Work out the finished part from the listing and answer in its coordinate system (mm). Face numbers are marked on the shaded views. A direction names the side the tool comes from. Coordinates: 2 decimals unless noted, no trailing zeros. Order: outer loops, then holes, each group sorted by start corner. A loop starts at its lowest first (then second) coordinate and runs counter-clockwise, first axis right, second up. Notation, with made-up numbers: M 44,-7.75 L 65,-7.75 A30 ccw 65,15.25 Z; hole C -18.75,13 d6. An arc over 180 degrees is marked long. Write item = value, one per line. Start each with the question number.
Q1. Straight lines are drawn through the part: line 1 along Y through (x, z) = (5, -7.5); line 2 along Z through (x, y) = (16, 13.5); line 3 along X through (y, z) = (4, -13). For each, find the intervals that lie inside material, in ascending order.
Q2. Find section B-B on z = -16. Give the vertices of the cut face in (x, y), and give its area (3 significant figures).
Q3. Find section A-A on y = 13.5. Give the vertices of the cut face in (x, z), and give its area (3 significant figures).
Q4. Determine the mould class of the marked faces 1, 2, 3 and 4 for opening direction X: released by +X, released by -X, zero draft, split by the parting line, or undercut.
Q5. A tool of negligible diameter and unlimited length cuts with its end or side. For the marked faces 5, 6 and 7, from which of +Z, -Z, +X, -X, +Y, -Y can it reach the whole face along a straight path? Write none if from no direction.
Q6. Each of these flat-tipped pins is pushed along its axis until it touches: P1, Ø5, axis at x = -6.5, z = -9, coming from the +Y side; P2, Ø5, axis at y = -2, z = 10, coming from the -X side; P3, Ø4, axis at y = -2.5, z = -10.5, coming from the +X side. Where does it stop, or does it pass through?
```python
from build123d import *

# Parameters (mm, degrees)
F4_D     = 4.2
F5_D     = 6.8
F6_D     = 6.6
F8_D     = 20
F8_DEPTH = 20
F8_TIP   = 6.0086061903


with BuildPart() as f2:
    # F1 (on Right) → F2 (revolve)
    with BuildSketch(Plane.YZ):
        Polygon((0, 0), (-16, 0), (-16, -12), (-12, -12), (-12, -30), (0, -30), align=None)
        Polygon((-22, 5), (-22, 0), (-16, 0), (0, 0), (0, 15), (-18, 15), (-18, 5), align=None)
    revolve(axis=Axis((0, 0, -7.8081190586), (0, 0, -1)))

    # F4 (through all)
    with Locations(Plane(origin=(0, 0, -30), x_dir=(1, 0, 0), z_dir=(0, 0, -1))):
        with Locations((4.0257674055, 6.3279694055)):
            Hole(F4_D / 2)

    # F5 (through all)
    with Locations(Plane(origin=(0, 0, -30), x_dir=(1, 0, 0), z_dir=(0, 0, -1))):
        with Locations((-3.2813517626, 2.2875162535)):
            Hole(F5_D / 2)

    # F6 (through all)
    with Locations(Plane(origin=(0, 0, -30), x_dir=(1, 0, 0), z_dir=(0, 0, -1))):
        with Locations((5.4357488604, -3.9169674911)):
            Hole(F6_D / 2)

    # F8
    with Locations(Plane.XY.offset(15)):
        with Locations((-3.2813517626, -2.2875162535)):
            Hole(F8_D / 2, depth=F8_DEPTH)
            with Locations((0, 0, -(F8_DEPTH + F8_TIP / 2))):  # 118° drill point
                Cone(0, F8_D / 2, F8_TIP, mode=Mode.SUBTRACT)


solid = f2.part
```
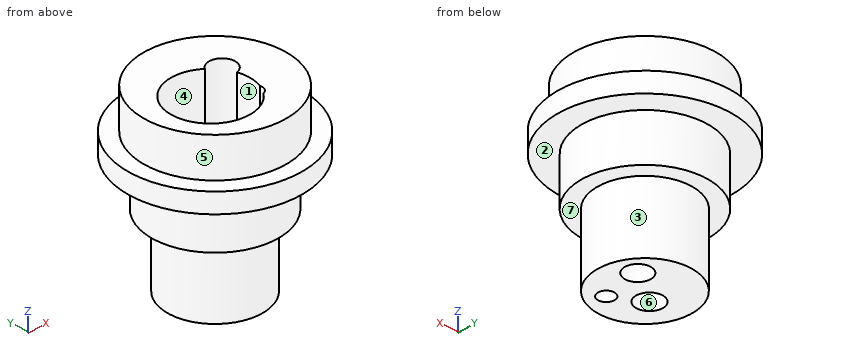
Findings below:
q1.line_1 = -15.2 to -8.19, -4.47 to 0.65, 7.19 to 15.2
q1.line_2 = 0 to 5
q1.line_3 = -11.31 to 2.14, 8.73 to 11.31
q2.outline = C 0,0 d24; hole C -3.28,-2.29 d6.8; hole C 4.03,-6.33 d4.2; hole C 5.44,3.92 d6.6
q2.area = 368 mm^2
q3.outline = M -17.37,0 L -8.59,0 L -8.59,-12 L 8.59,-12 L 8.59,0 L 17.37,0 L 17.37,5 L 11.91,5 L 11.91,15 L -11.91,15 L -11.91,5 L -17.37,5 Z
q3.area = 618 mm^2
q4.face_1 = undercut
q4.face_2 = zero draft
q4.face_3 = split by the parting line
q4.face_4 = undercut
q5.face_5 = +Z
q5.face_6 = +Z, -Z
q5.face_7 = -Z
q6.P1 = 15.49
q6.P2 = -18
q6.P3 = 15.99
